```python
from build123d import *

# Parameters (mm, degrees)
BOSS_EXTRUDE1_DEPTH = 26.924


with BuildPart() as part:
    # Sketch1 → Boss-Extrude1 (new, symmetric)
    with BuildSketch(Plane(origin=(0, 0, 0), x_dir=(1, 0, 0), z_dir=(0, 1, 0))):
        Polygon((-16.038691669, 65.646737994), (0, 65.646737994), (0, -45.132132371), (89.518279083, -45.132132371), (89.518279083, -57.813888574), (-16.038691669, -57.813888574), (-16.038691669, -45.132132371), align=None)
    boss_extrude1 = extrude(amount=BOSS_EXTRUDE1_DEPTH, both=True)

    # Mirror1: Boss-Extrude1 across plane
    add(boss_extrude1.mirror(Plane(origin=(-16.038691669, 26.924, -65.646737994), x_dir=(1, 0, 0), z_dir=(0, 0, 1))))


solid = part.part
```
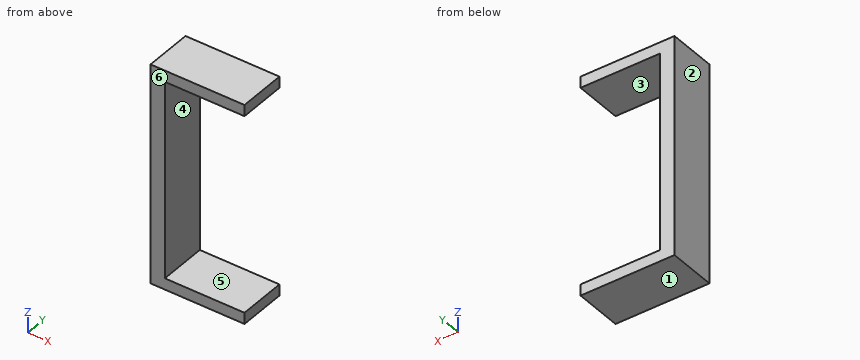
Could you check a few things on this model? Use its own coordinates, in mm. Face numbers are marked on the shaded views. A direction names the side the tool comes from. Coordinates: 2 decimals unless noted, no trailing zeros. Write each loop counter-clockwise with the first axis right and the second up, starting at its lowest first coordinate (ties: lowest second). Pieces come first, ordered by that corner, then holes. Notation, with made-up numbers: (37, -31.75) -> (49, -31.75) arc R17 ccw to (49, -20.75) -> close; hole circle Ø11 at (-33.5, -2). An arc over 180 degrees is marked (long way). One line per question, with ' | ' between items. Start each with the question number.
1. Thinking about a two-plate mould opening in Z: for the marked faces 1, 2, 3 and 4, which applies, pulls with the +Z half, pulls with the -Z half, needs draft (parallel to the pull), parting line crosses it, or undercut?
2. If we section it at C-C (z = -115): Please give me the cut outline in (x, y), and give its area (3 significant figures).
3. Please list where these lines run through material, in increasing order: line 1 along Z through (x, y) = (45, -6); line 2 along X through (y, z) = (-0.5, -117).
4. Will this pin go through, and if not, where does the flat tip stop? P1, Ø1, axis at y = -5.5, z = 30.5, coming from the +X side.
5. If we section it at B-B (y = 15): Please give me the cut outline in (x, z).
6. If we section it at A-A (x = 20.5): Please give me the cut outline in (y, z), and give its area (3 significant figures).
7. For the marked faces 5 and 6, which set-ups out of +Z, -Z, +X, -X, +Y, -Y let a thin tool reach every point of the face, with its end or its side?
Return value:
1) face 1: pulls with the -Z half | face 2: needs draft | face 3: undercut | face 4: undercut
2) outline: (-16.04, -26.92) -> (0, -26.92) -> (0, 26.92) -> (-16.04, 26.92) -> close | area: 864 mm²
3) line 1: z = -189.11 to -176.43, 45.13 to 57.81 | line 2: x = -16.04 to 0
4) P1: stops at x = 0
5) outline: (-16.04, -189.11) -> (89.52, -189.11) -> (89.52, -176.43) -> (0, -176.43) -> (0, 45.13) -> (89.52, 45.13) -> (89.52, 57.81) -> (-16.04, 57.81) -> close
6) outline: (-26.92, -189.11) -> (26.92, -189.11) -> (26.92, -176.43) -> (-26.92, -176.43) -> close; (-26.92, 45.13) -> (26.92, 45.13) -> (26.92, 57.81) -> (-26.92, 57.81) -> close | area: 1,370 mm²
7) face 5: +X, +Y, -Y | face 6: +Z, -Z, +X, -X, -Y
